from build123d import *

# Parameters (mm, degrees)
SKETCH1_R           = 12.1
SKETCH1_W           = 20.2
SKETCH1_H           = 40.2
BASE_PLATE_DEPTH    = 4
FILLET1_R           = 1
FILLET2_R           = 2
SKETCH2_R           = 1.875
CUT_EXTRUDE1_DEPTH  = 78.256779638
SKETCH3_W           = 4
SKETCH3_H           = 40.2
BOSS_EXTRUDE1_DEPTH = 28.2
CUT_EXTRUDE2_DEPTH  = 78.256779638
FILLET3_R           = 1
FILLET5_R           = 0.35


with BuildPart() as part:
    # Sketch1 → Base Plate (new body)
    with BuildSketch(Plane.XY):
        with BuildLine():
            Line((-18.1, -62), (-18.1, 75))
            Line((-18.1, 75), (18.1, 75))
            Line((18.1, 75), (18.1, -62))
            ThreePointArc((18.1, -62), (14.292388155, -71.192388155), (5.1, -75))
            Line((5.1, -75), (-5.1, -75))
            ThreePointArc((-5.1, -75), (-14.292388155, -71.192388155), (-18.1, -62))
        make_face()
        with Locations((0, -48.3)):
            Circle(SKETCH1_R, mode=Mode.SUBTRACT)
        Polygon((-10.1, 28.1), (4.1, 28.1), (-10.1, 67), align=None, mode=Mode.SUBTRACT)
        Rectangle(SKETCH1_W, SKETCH1_H, mode=Mode.SUBTRACT)
        Polygon((10.1, 67), (-4.1, 67), (10.1, 28.1), align=None, mode=Mode.SUBTRACT)
    extrude(amount=BASE_PLATE_DEPTH)

    # Fillet1
    fillet1_edges = [part.edges().sort_by_distance(p)[0] for p in [
        (10.1, 28.1, 2),
        (10.1, 67, 2),
        (-4.1, 67, 2),
        (-10.1, 67, 2),
        (-10.1, 28.1, 2),
        (4.1, 28.1, 2),
    ]]
    fillet(fillet1_edges, radius=FILLET1_R)

    # Fillet2
    fillet2_edges = [part.edges().sort_by_distance(p)[0] for p in [
        (-18.1, 75, 2),
        (18.1, 75, 2),
    ]]
    fillet(fillet2_edges, radius=FILLET2_R)

    # Sketch2 → Cut-Extrude1 (cut, through all)
    with BuildSketch(Plane.XY.offset(4)):
        with Locations((5, 24.75)):
            Circle(SKETCH2_R)
        with Locations((-5, 24.75)):
            Circle(SKETCH2_R)
        with Locations(Location((-5, -24.75, 0), (0, 0, 180))):
            Circle(SKETCH2_R)
        with Locations(Location((5, -24.75, 0), (0, 0, 180))):
            Circle(SKETCH2_R)
        with Locations((13.4, 24.75)):
            Circle(SKETCH2_R)
        with Locations(Location((-13.4, 24.75, 0), (0, 0, 180))):
            Circle(SKETCH2_R)
        with Locations(Location((13.4, -24.75, 0), (0, 0, 180))):
            Circle(SKETCH2_R)
        with Locations((-13.4, -24.75)):
            Circle(SKETCH2_R)
        with Locations((13.4, 70.3)):
            Circle(SKETCH2_R)
        with Locations(Location((-13.4, 70.3, 0), (0, 0, 180))):
            Circle(SKETCH2_R)
        with Locations((0, -69.3)):
            Circle(SKETCH2_R)
    extrude(amount=-CUT_EXTRUDE1_DEPTH, mode=Mode.SUBTRACT)

    # Sketch3 → Boss-Extrude1 (add, through all)
    with BuildSketch(Plane.ZY.offset(-10.1)):
        with Locations((2, 0)):
            Rectangle(SKETCH3_W, SKETCH3_H)
    extrude(amount=BOSS_EXTRUDE1_DEPTH)

    # Sketch4 → Cut-Extrude2 (cut, through all)
    with BuildSketch(Plane.XY.offset(4)):
        Polygon((-10.1, 20.1), (-10.1, -20.1), (3.9, -20.1), align=None)
        Polygon((-3.9, 20.1), (10.1, 20.1), (10.1, -20.1), align=None)
    extrude(amount=-CUT_EXTRUDE2_DEPTH, mode=Mode.SUBTRACT)

    # Fillet3
    fillet3_edges = [part.edges().sort_by_distance(p)[0] for p in [
        (10.1, -20.1, 2),
        (-3.9, 20.1, 2),
        (10.1, 20.1, 2),
        (-10.1, 20.1, 2),
        (3.9, -20.1, 2),
        (-10.1, -20.1, 2),
    ]]
    fillet(fillet3_edges, radius=FILLET3_R)

    # Fillet5
    fillet5_edges = [part.edges().sort_by_distance(p)[0] for p in [
        (17.514213562, 74.414213562, 4),
        (-17.514213562, 74.414213562, 4),
        (-14.292388155, -71.192388155, 4),
        (0, -75, 4),
        (14.292388155, -71.192388155, 4),
        (-12.1, -48.3, 0),
        (-12.1, -48.3, 4),
        (18.1, 5.5, 4),
        (14.292388155, -71.192388155, 0),
        (0, -75, 0),
        (-14.292388155, -71.192388155, 0),
        (18.1, 5.5, 0),
        (-18.1, 5.5, 0),
        (-18.1, 5.5, 4),
        (0, 75, 0),
        (17.514213562, 74.414213562, 0),
        (-17.514213562, 74.414213562, 0),
        (0, 75, 4),
    ]]
    fillet(fillet5_edges, radius=FILLET5_R)


solid = part.part
Could you check a few things on this model? Use its own coordinates, in mm. A direction names the side the tool comes from. Give positions to 0.01 mm unless a question says otherwise; leave off trailing zeros. Order: outer loops, then holes, each group sorted by start corner. A loop starts at its lowest first (then second) coordinate and runs counter-clockwise, first axis right, second up.
1. Suppose I cut it at B-B (y = 5). List the corners of the cut face in (x, z) for me, plus the area to 3 significant figures.
2. We'd pull the mould along Y, two halves only. Please class faces 1 (the flat face through (0, 1, 4)), 2 (the flat face through (0, 75, 2)), 3 (the cylindrical face through (-12.99, 72.13, 2.03)): pulls with the +Y half, pulls with the -Y half, needs draft (parallel to the pull), parting line crosses it, or undercut.
3. Will these pins go through, and if not, where does the flat tip stop? P1, Ø2, axis at x = -13.5, z = 2, coming from the -Y side; P2, Ø4.5, axis at x = 13.4, y = -24.75, coming from the +Z side; P3, Ø1, axis at x = 9.5, z = 0.5, coming from the -Y side.
4. Suppose I cut it at A-A (y = 24.75). List the corners of the cut face in (x, z) for me (3 decimals).
5. I need wall thicknesses on L1, parallel to X at y = 70.3, z = 1.3 (3 decimals); L2, parallel to X at y = -8, z = 1.4; L3, parallel to Y at x = -10, z = 3. Which ranges of each line are inside material? Lowest first, please.
6. For faces 4 (the flat face through (-18.1, 6, 2)), 5 (the flat face through (-3, -20.1, 2)), which set-ups out of +Z, -Z, +X, -X, +Y, -Y let a thin tool reach every point of the face, with its end or its side?
7. Suppose I cut it at C-C (z = 2.2). Give the number of separate pieces and of enclosed holes in the cut face, plus the area to 3 significant figures.
Solved:
1. outline: (-18.1, 0.35) arc R0.35 ccw to (-17.75, 0) - (-10.1, 0) - (-10.1, 4) - (-17.75, 4) arc R0.35 ccw to (-18.1, 3.65) - close; (-4.84, 0) - (1.36, 0) - (1.36, 4) - (-4.84, 4) - close; (10.1, 0) - (17.75, 0) arc R0.35 ccw to (18.1, 0.35) - (18.1, 3.65) arc R0.35 ccw to (17.75, 4) - (10.1, 4) - close
1. area: 88.7 mm2
2. face 1: needs draft
2. face 2: pulls with the +Y half
2. face 3: undercut
3. P1: stops at y = -72.69
3. P2: stops at z = 4
3. P3: stops at y = -74.4
4. outline: (-18.1, 0.35) arc R0.35 ccw to (-17.75, 0) - (-15.275, 0) - (-15.275, 4) - (-17.75, 4) arc R0.35 ccw to (-18.1, 3.65) - close; (-11.525, 0) - (-6.875, 0) - (-6.875, 4) - (-11.525, 4) - close; (-3.125, 0) - (3.125, 0) - (3.125, 4) - (-3.125, 4) - close; (6.875, 0) - (11.525, 0) - (11.525, 4) - (6.875, 4) - close; (15.275, 0) - (17.75, 0) arc R0.35 ccw to (18.1, 0.35) - (18.1, 3.65) arc R0.35 ccw to (17.75, 4) - (15.275, 4) - close
5. L1: x = -18.1 to -15.275, -11.525 to 11.525, 15.275 to 18.1
5. L2: x = -18.1 to -10.1, -0.31 to 5.89, 10.1 to 18.1
5. L3: y = -74.04 to -55.11, -41.49 to -19.54, 14.62 to 28.66, 61.78 to 75
6. face 4: +Z, -Z, -X, +Y, -Y
6. face 5: +Z, -Z
7. separate pieces: 1
7. enclosed holes: 16
7. area: 3,680 mm2
